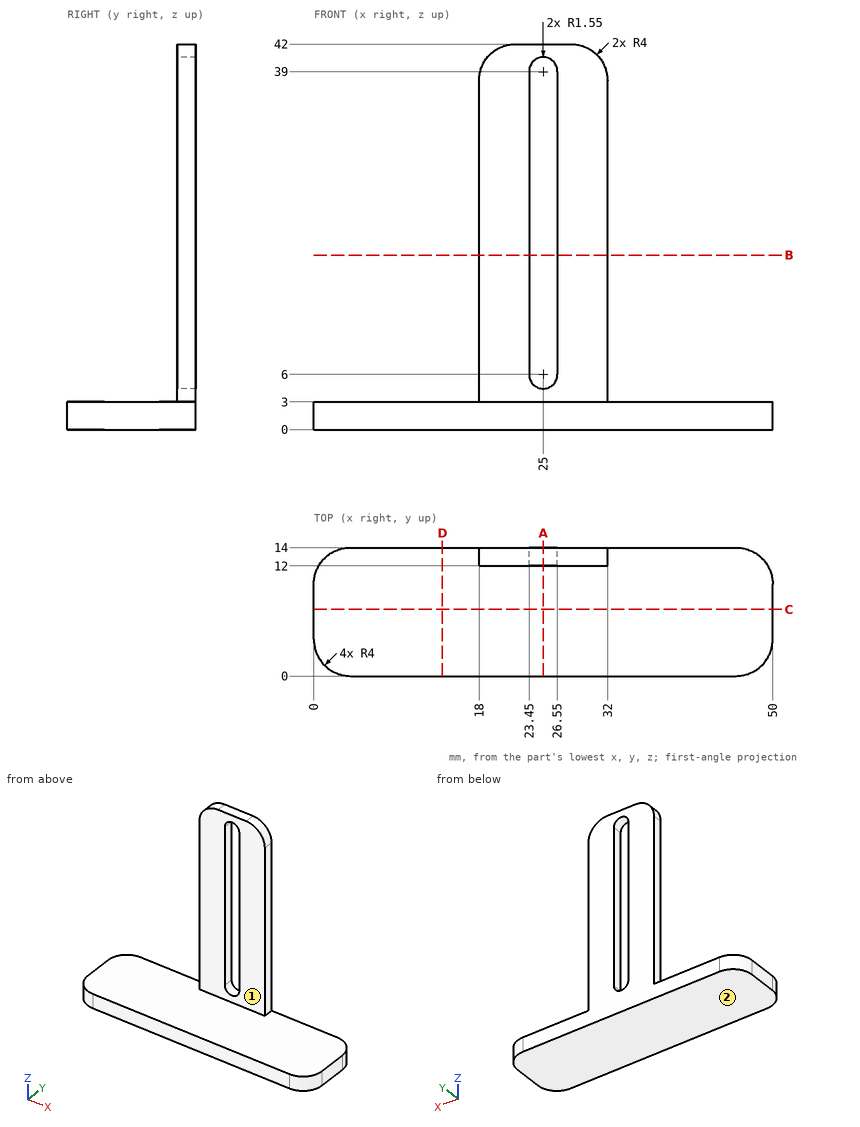
Drawing for the job (mm, zero at the part's lowest x, y, z). A direction names the side the tool comes from. Give positions to 0.01 mm unless a question says otherwise; leave off trailing zeros. Write each loop counter-clockwise with the first axis right and the second up, starting at its lowest first coordinate (ties: lowest second). Pieces come first, ordered by that corner, then holes. Notation, with made-up numbers: M -32,52.5 L 0,52.5 A28 cw 0,78.5 Z; hole C 65.5,22 d1. An arc over 180 degrees is marked long. Return JSON: item names as keys, results as strings. Group by question number.
(1) Band-saw the part on D-D (x = 14). Give the cut face in (y, z), and give its area (3 significant figures).
(2) 3-axis set-ups, long thin cutter, end or side, ignore diameter. For the marked faces 1 and 2: which of +Z, -Z, +X, -X, +Y, -Y reach the whole face in a straight line?
(3) Drill centre lines: L1, parallel to Z at x = 22.5, y = 7; L2, parallel to Y at x = 22, z = 10; L3, parallel to Z at x = 21.5, y = 12.75. Where is each one in solid material? Low to high. Write a range as [from, to].
(4) Flat gauge pins, fed straight in: pin 1 Ø6 at (x, z) = (26.5, 36.5) entering from -Y; pin 2 Ø5 at (x, y) = (23.5, 7.5) entering from +Z; pin 3 Ø6 at (x, z) = (38, 7.5) entering from +Y; pin 4 Ø2 at (y, z) = (12.5, 22) entering from +X. Where does each tip first touch, or does it go through?
(5) Band-saw the part on C-C (y = 7.25). Give the cut face in (x, z).
(6) Band-saw the part on B-B (z = 19). Give the cut face in (x, y).
(7) Band-saw the part on A-A (x = 25). Give the cut face in (y, z), and give its area (3 significant figures).
Entries:
{
 "1": {"outline": "M 0,0 L 14,0 L 14,3 L 0,3 Z", "area": "42.0 mm^2"},
 "2": {"face 1": "+Z, +X, -X, -Y", "face 2": "-Z, +X, -X, +Y, -Y"},
 "3": {"L1": "z = [0, 3]", "L2": "y = [12, 14]", "L3": "z = [0, 41.97]"},
 "4": {"pin 1": "stops at y = 12", "pin 2": "stops at z = 3", "pin 3": "passes through", "pin 4": "stops at x = 32"},
 "5": {"outline": "M 0,0 L 50,0 L 50,3 L 0,3 Z"},
 "6": {"outline": "M 18,12 L 23.45,12 L 23.45,14 L 18,14 Z; M 26.55,12 L 32,12 L 32,14 L 26.55,14 Z"},
 "7": {"outline": "M 0,0 L 14,0 L 14,4.45 L 12,4.45 L 12,3 L 0,3 Z; M 12,40.55 L 14,40.55 L 14,42 L 12,42 Z", "area": "47.8 mm^2"}
}
